```python
from build123d import *

# Parameters (mm, degrees)
BOSS_EXTRUDE1_DEPTH  = 3.175
M6_CLEARANCE_HOLE1_D = 6.6
FILLET1_R            = 3.175


with BuildPart() as part:
    # Sketch1 → Boss-Extrude1 (new body)
    with BuildSketch(Plane.XY):
        Polygon((-141.015921324, 133.528527902), (-133.395921324, 133.528527902), (-133.395921324, 118.528527902), (-141.015921324, 118.528527902), (-145.065921324, 118.528527902), (-145.065921324, 70.028527902), (-160.065921324, 70.028527902), (-160.065921324, 133.528527902), align=None)
    extrude(amount=BOSS_EXTRUDE1_DEPTH)

    # M6 Clearance Hole1 (through all)
    with Locations(Plane.XY.offset(3.175)):
        with Locations((-141.015921324, 126.028527902), (-152.565921324, 77.648527902)):
            Hole(M6_CLEARANCE_HOLE1_D / 2)

    # Fillet1
    fillet1_edges = [part.edges().sort_by_distance(p)[0] for p in [
        (-145.065921324, 118.528527902, 1.5875),
        (-145.065921324, 70.028527902, 1.5875),
        (-160.065921324, 70.028527902, 1.5875),
        (-160.065921324, 133.528527902, 1.5875),
        (-133.395921324, 133.528527902, 1.5875),
        (-133.395921324, 118.528527902, 1.5875),
    ]]
    fillet(fillet1_edges, radius=FILLET1_R)


solid = part.part
```
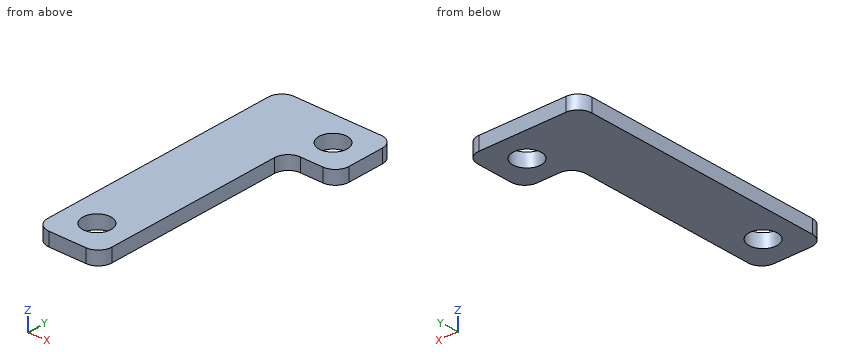
Read the model definition and answer for the solid it produces. Units are mm, in the model's axes. Coordinates: 2 decimals unless noted, no trailing zeros. Loops run counter-clockwise (first coordinate to the right, second up) from the corner with the lowest first, then second, coordinate; pieces in that order, holes last. Notation, with made-up numbers: (14.25, -19.75) -> (27.25, -19.75) arc R22 ccw to (27.25, 3.25) -> close; hole circle Ø1 at (44, -38.5). An arc over 180 degrees is marked (long way). Return JSON: item names as keys, results as strings.
Item 1: Find section A-A (x = -139.75). Determine the outline of the cut face in (y, z) (3 decimals), plus the area to 3 significant figures.
Answers:
{"outline": "(118.529, 0) -> (122.981, 0) -> (122.981, 3.175) -> (118.529, 3.175) -> close; (129.076, 0) -> (133.529, 0) -> (133.529, 3.175) -> (129.076, 3.175) -> close", "area": "28.3 mm2"}
Item 2: Find the intervals of material crossed by probe 1 along Y at (x, z) = (-141, 2.6); probe 2 along X at (y, z) = (80, 2.8); probe 3 along Y at (x, z) = (-137, 0.55), in increasing order.
Answers:
{"probe 1": "y = 118.53 to 122.73, 129.33 to 133.53", "probe 2": "x = -160.07 to -154.88, -150.25 to -145.07", "probe 3": "y = 118.53 to 133.53"}
Item 3: Find section C-C (z = 0.8). Determine the outline of the cut face in (x, y) (3 decimals), plus the area to 3 significant figures.
Answers:
{"outline": "(-160.066, 73.204) arc R3.175 ccw to (-156.891, 70.029) -> (-148.241, 70.029) arc R3.175 ccw to (-145.066, 73.204) -> (-145.066, 115.354) arc R3.175 cw to (-141.891, 118.529) -> (-136.571, 118.529) arc R3.175 ccw to (-133.396, 121.704) -> (-133.396, 130.354) arc R3.175 ccw to (-136.571, 133.529) -> (-156.891, 133.529) arc R3.175 ccw to (-160.066, 130.354) -> close; hole circle Ø6.6 at (-152.566, 77.649); hole circle Ø6.6 at (-141.016, 126.029)", "area": "1,050 mm2"}
Item 4: Find section D-D (y = 95). Determine the outline of the cut face in (x, z) (3 decimals).
Answers:
{"outline": "(-160.066, 0) -> (-145.066, 0) -> (-145.066, 3.175) -> (-160.066, 3.175) -> close"}
Item 5: Flat-ended cylindrical pins translate along their axes: P1, Ø1.5, axis at x = -147, z = 1, coming from the -Y side; P2, Ø5.5, axis at x = -152.57, y = 77.65, coming from the -Z side. Find the tip coordinate at first contact, or state that the pin passes through.
Answers:
{"P1": "stops at y = 70.07", "P2": "passes through"}
Item 6: Find section B-B (y = 76). Determine the outline of the cut face in (x, z) (3 decimals).
Answers:
{"outline": "(-160.066, 0) -> (-155.425, 0) -> (-155.425, 3.175) -> (-160.066, 3.175) -> close; (-149.707, 0) -> (-145.066, 0) -> (-145.066, 3.175) -> (-149.707, 3.175) -> close"}
